from build123d import *

# Parameters (mm, degrees)
SKETCH1_W               = 840
SKETCH1_H               = 501
SKETCH1_R               = 5
BOSS_EXTRUDE1_DEPTH     = 2.4
SKETCH2_W               = 112
SKETCH2_H               = 30
CUT_EXTRUDE1_DEPTH      = 34
MIRROR2_COPY_1_SKETCH_W = 112
MIRROR2_COPY_1_SKETCH_H = 30
MIRROR2_COPY_1_DEPTH    = 34


with BuildPart() as part:
    # Sketch1 → Boss-Extrude1 (new body)
    with BuildSketch(Plane.XY):
        with Locations((420, 250.5)):
            Rectangle(SKETCH1_W, SKETCH1_H)
        with Locations((825.625, 486.625)):
            Circle(SKETCH1_R, mode=Mode.SUBTRACT)
        with Locations((14.375, 14.375)):
            Circle(SKETCH1_R, mode=Mode.SUBTRACT)
        with Locations((14.375, 486.625)):
            Circle(SKETCH1_R, mode=Mode.SUBTRACT)
        with Locations((825.625, 14.375)):
            Circle(SKETCH1_R, mode=Mode.SUBTRACT)
    extrude(amount=BOSS_EXTRUDE1_DEPTH)

    # Sketch2 → Cut-Extrude1 (cut)
    with BuildSketch(Plane.XY.offset(2.4)):
        with Locations((90.32, 101.47)):
            Rectangle(SKETCH2_W, SKETCH2_H)
    cut_extrude1 = extrude(amount=-CUT_EXTRUDE1_DEPTH, mode=Mode.SUBTRACT)

    # Mirror1: Cut-Extrude1 across plane
    add(cut_extrude1.mirror(Plane(origin=(420, 0, 0), x_dir=(0, 0, 1), z_dir=(1, 0, 0))), mode=Mode.SUBTRACT)

    # Mirror2: Cut-Extrude1 across plane
    add(cut_extrude1.mirror(Plane(origin=(0, 250.5, 0), x_dir=(0, 0, 1), z_dir=(0, -1, 0))), mode=Mode.SUBTRACT)

    # Mirror2 copy 1 sketch → Mirror2 copy 1 (cut)
    with BuildSketch(Plane(origin=(840, 501, 2.4), x_dir=(-1, 0, 0), z_dir=(0, 0, 1))):
        with Locations((90.32, 101.47)):
            Rectangle(MIRROR2_COPY_1_SKETCH_W, MIRROR2_COPY_1_SKETCH_H)
    extrude(amount=-MIRROR2_COPY_1_DEPTH, mode=Mode.SUBTRACT)


solid = part.part
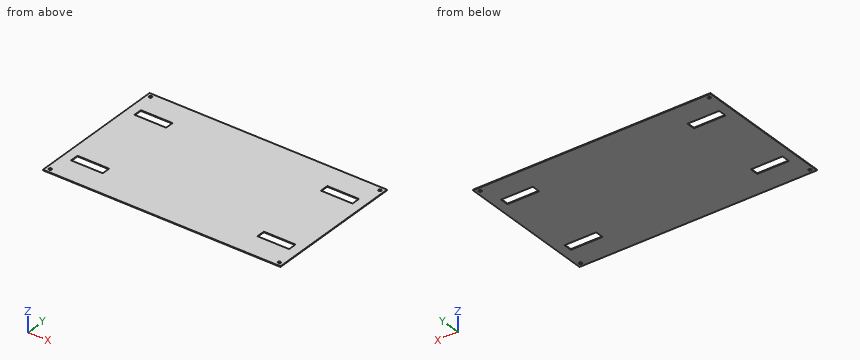
Geometry: final body of the model. Coordinates: model frame, mm. Round coordinates to 2 decimals unless told otherwise and drop trailing zeros. Write item = value, one per line.
Item 1: Material intervals for line 1 along X through (y, z) = (400.5, 1.5), sorted ascending. Write a range as [from, to].
Findings:
line_1 = [0, 34.32], [146.32, 693.68], [805.68, 840]
Item 2: Section query A-A on z = 1.3. State how many separate pieces and enclosed holes the cut face has, then the cut area to 3 significant figures.
Findings:
separate_pieces = 1
enclosed_holes = 8
area = 407,000 mm^2
Item 3: Pin query (flat end, axial travel): P1, Ø9, axis at x = 14.375, y = 486.625, coming from the -Z side. Return the tip coordinate at first contact, or that it passes through.
Findings:
P1 = through
